```python
from build123d import *
from build123d.topology import SkipClean

# Parameters (mm, degrees)
SKETCH1_R           = 40
BOSS_EXTRUDE1_DEPTH = 40
SKETCH2_R           = 38
CUT_EXTRUDE1_DEPTH  = 38
CUT_EXTRUDE2_DEPTH  = 38
SKETCH4_R           = 5
CUT_EXTRUDE3_DEPTH  = 38
SKETCH6_R           = 2
BOSS_EXTRUDE2_DEPTH = 2
BOSS_EXTRUDE3_START = 10
SKETCH9_R           = 40
SKETCH9_R_2         = 38
BOSS_EXTRUDE3_DEPTH = 10
BOSS_EXTRUDE4_DEPTH = 32
CUT_EXTRUDE4_DEPTH  = 30
FILLET1_R           = 0.25
SKETCH13_R          = 3
CUT_EXTRUDE5_DEPTH  = 10


with BuildPart() as part:
    # Sketch1 → Boss-Extrude1 (new body)
    with BuildSketch(Plane(origin=(0, 0, 0), x_dir=(1, 0, 0), z_dir=(0, 1, 0))):
        with Locations(Location((0, 0, 0), (0, 0, 270))):
            Circle(SKETCH1_R)
    extrude(amount=BOSS_EXTRUDE1_DEPTH)

    # Sketch2 → Cut-Extrude1 (cut)
    with BuildSketch(Plane(origin=(0, 40, 0), x_dir=(1, 0, 0), z_dir=(0, 1, 0))):
        with Locations(Location((0, 0, 0), (0, 0, 270))):
            Circle(SKETCH2_R)
    extrude(amount=-CUT_EXTRUDE1_DEPTH, mode=Mode.SUBTRACT)

    # Sketch3 → Cut-Extrude2 (cut)
    with SkipClean():  # the faces are left unmerged after this step: merging them gives an invalid solid
        with BuildSketch(Plane(origin=(0, 2, 0), x_dir=(1, 0, 0), z_dir=(0, 1, 0))):
            with BuildLine():
                ThreePointArc((-14.076066703, -35.296803626), (0, -24.534862453), (14.076066703, -35.296803626))
                ThreePointArc((14.076066703, -35.296803626), (0, -38), (-14.076066703, -35.296803626))
            make_face()
        extrude(amount=-CUT_EXTRUDE2_DEPTH, mode=Mode.SUBTRACT)

    # Sketch4 → Cut-Extrude3 (cut)
    with SkipClean():  # the faces are left unmerged after this step: merging them gives an invalid solid
        with BuildSketch(Plane(origin=(0, 2, 0), x_dir=(1, 0, 0), z_dir=(0, 1, 0))):
            with Locations(Location((0, 0, 0), (0, 0, 270))):
                Circle(SKETCH4_R)
        extrude(amount=-CUT_EXTRUDE3_DEPTH, mode=Mode.SUBTRACT)

    # Sketch6 → Boss-Extrude2 (add)
    with SkipClean():  # the faces are left unmerged after this step: merging them gives an invalid solid
        with BuildSketch(Plane.XZ):
            with Locations(Location((-20, 0, 0), (0, 0, 90))):
                Circle(SKETCH6_R)
            with Locations(Location((20, 0, 0), (0, 0, 90))):
                Circle(SKETCH6_R)
        extrude(amount=BOSS_EXTRUDE2_DEPTH)

    # Sketch9 → Boss-Extrude3 (add)
    with SkipClean():  # the faces are left unmerged after this step: merging them gives an invalid solid
        with BuildSketch(Plane(origin=(0, 40, 0), x_dir=(1, 0, 0), z_dir=(0, 1, 0)).offset(BOSS_EXTRUDE3_START)):
            with Locations(Location((0, 0, 0), (0, 0, 270))):
                Circle(SKETCH9_R)
            with Locations(Location((0, 0, 0), (0, 0, 270))):
                Circle(SKETCH9_R_2, mode=Mode.SUBTRACT)
        extrude(amount=-BOSS_EXTRUDE3_DEPTH)

    # Sketch10 → Boss-Extrude4 (add)
    with SkipClean():  # the faces are left unmerged after this step: merging them gives an invalid solid
        with BuildSketch(Plane(origin=(0, 50, 0), x_dir=(1, 0, 0), z_dir=(0, 1, 0))):
            Polygon((0, -38), (10, -38), (10, -48), (-10, -48), (-10, -38), align=None)
        extrude(amount=-BOSS_EXTRUDE4_DEPTH)

    # Sketch11 → Cut-Extrude4 (cut)
    with SkipClean():  # the faces are left unmerged after this step: merging them gives an invalid solid
        with BuildSketch(Plane(origin=(0, 50, 0), x_dir=(1, 0, 0), z_dir=(0, 1, 0))):
            Polygon((-3, -36.864916731), (3, -36.864916731), (3, -41.364916731), (6.5, -41.364916731), (6.5, -46.364916731), (-6.5, -46.364916731), (-6.5, -41.364916731), (-3, -41.364916731), align=None)
        extrude(amount=-CUT_EXTRUDE4_DEPTH, mode=Mode.SUBTRACT)

    # Fillet1
    fillet1_edges = [part.edges().sort_by_distance(p)[0] for p in [
        (-3, 35, 41.364916731),
        (6.5, 35, 46.364916731),
        (-6.5, 35, 46.364916731),
        (-6.5, 35, 41.364916731),
        (3, 35, 41.364916731),
        (6.5, 35, 41.364916731),
    ]]
    fillet(fillet1_edges, radius=FILLET1_R)

    # Sketch13 → Cut-Extrude5 (cut)
    with BuildSketch(Plane.XZ):
        with Locations(Location((-30, 0, 0), (0, 0, 270))):
            Circle(SKETCH13_R)
        with Locations(Location((30, 0, 0), (0, 0, 270))):
            Circle(SKETCH13_R)
    extrude(amount=-CUT_EXTRUDE5_DEPTH, mode=Mode.SUBTRACT)


solid = part.part
```
Geometry check sheet. Reference: the model listing, model coordinates, mm. A direction names the side the tool comes from. Round coordinates to 2 decimals unless told otherwise and drop trailing zeros. Loops run counter-clockwise (first coordinate to the right, second up) from the corner with the lowest first, then second, coordinate; pieces in that order, holes last. Notation, with made-up numbers: (-39.75, 6.5) - (10.25, 6.5) arc R20 ccw to (10.25, 36.5) - close; hole circle Ø6 at (-27.5, 86). An arc over 180 degrees is marked (long way). Write item = value, one per line. Start each with the question number.
1. Thickness scan on line 1 (X direction, y = 0.7, z = 0); line 2 (Z direction, x = 0, y = 47); line 3 (X direction, y = 47.5, z = 0). Record the ranges inside material, lowest first.
2. Section check A-A on z = 0. Enter the section's corners in (x, y), then the cut area to 3 significant figures.
3. Section check C-C on y = 22. Enter the section's corners in (x, z), then the cut area to 3 significant figures.
4. Set-up check for faces 1 (the face through (18, -1, 0)), 2 (the face through (-10, 34, 43)), 3 (the face through (-0.267, 1.014, 24.537)), 4 (the face through (3, 35, 39)), 5 (the face through (10, 34, 43)): record each of +Z, -Z, +X, -X, +Y, -Y from which the full face is reachable in a straight line by a thin tool's end or side.
5. Depth check by flat-ended pin: pin 1 (1 mm diameter, centred on x = -16, y = 13, fed in from +Z); pin 2 (1.5 mm diameter, centred on x = 21, z = 11.5, fed in from +Y); pin 3 (10 mm diameter, centred on y = 39.5, z = 13, fed in from -X); pin 4 (9.5 mm diameter, centred on x = 3, z = 41.5, fed in from +Y). Enter the tip coordinate at first touch or a pass-through.
6. Section check B-B on x = -11.5. Enter the section's corners in (y, z).
7. Section check D-D on x = 20. Enter the section's corners in (y, z), then the cut area to 3 significant figures.
Working result:
q1.line_1 = -40 to -33, -27 to -5, 5 to 27, 33 to 40
q1.line_2 = -40 to -38, 46.36 to 48
q1.line_3 = -40 to -38, 38 to 40
q2.outline = (-40, 0) - (-33, 0) - (-33, 2) - (-38, 2) - (-38, 50) - (-40, 50) - close; (-27, 0) - (-22, 0) - (-22, -2) - (-18, -2) - (-18, 0) - (-5, 0) - (-5, 2) - (-27, 2) - close; (5, 0) - (18, 0) - (18, -2) - (22, -2) - (22, 0) - (27, 0) - (27, 2) - (5, 2) - close; (33, 0) - (40, 0) - (40, 50) - (38, 50) - (38, 2) - (33, 2) - close
q2.area = 324 mm^2
q3.outline = (-10, 38.73) arc R40 ccw (long way) to (10, 38.73) - (10, 48) - (-10, 48) - close; hole (-6.5, 41.61) arc R0.25 ccw to (-6.25, 41.36) - (-3.25, 41.36) arc R0.25 cw to (-3, 41.11) - (-3, 37.88) arc R38 ccw (long way) to (3, 37.88) - (3, 41.11) arc R0.25 cw to (3.25, 41.36) - (6.25, 41.36) arc R0.25 ccw to (6.5, 41.61) - (6.5, 46.11) arc R0.25 ccw to (6.25, 46.36) - (-6.25, 46.36) arc R0.25 ccw to (-6.5, 46.11) - close
q3.area = 573 mm^2
q4.face_1 = -Y
q4.face_2 = +Z, -X, +Y, -Y
q4.face_3 = +Y, -Y
q4.face_4 = +Y
q4.face_5 = +Z, +X, +Y, -Y
q5.pin_1 = 36.87
q5.pin_2 = 2
q5.pin_3 = -39.19
q5.pin_4 = 50
q6.outline = (0, -38.31) - (50, -38.31) - (50, -36.22) - (2, -36.22) - (2, 30.15) - (0, 30.15) - close; (0, 36.22) - (50, 36.22) - (50, 38.31) - (0, 38.31) - close
q7.outline = (-2, -2) - (0, -2) - (0, -34.64) - (50, -34.64) - (50, -32.31) - (2, -32.31) - (2, 32.31) - (50, 32.31) - (50, 34.64) - (0, 34.64) - (0, 2) - (-2, 2) - close
q7.area = 370 mm^2
